Autodesk Inventor part; units mm, degrees
ref_plane "YZ Plane" through (0, 0, 0) normal (1, 0, 0) x (0, 1, 0)
ref_plane "XZ Plane" through (0, 0, 0) normal (0, 1, 0) x (-1, 0, 0)
ref_plane "XY Plane" through (0, 0, 0) normal (0, 0, 1) x (1, 0, 0)
sketch "Sketch1" plane through (0, 0, 0) normal (0, 0, 1) x (1, 0, 0)
  line L0 (-10, 4.2062) -> (5, 4.2062) construction
  line L1 (-10, -0.7938) -> (5, -0.7938)
  line L2 (5, 9.2062) -> (-10, 9.2062)
  arc A0 (-10, 9.2062) -> (-10, -0.7938) centre (-10, 4.2062) ccw
  arc A1 (5, -0.7938) -> (5, 9.2062) centre (5, 4.2062) ccw
  circle A2 centre (-2.5, 4.2062) radius 2.5
  point P0 (0, 0)
  dimension "d0" = 10
  dimension "d1" = 5
  dimension "d11" = 15
extrude "Extrusion3" add sketch "Sketch1" along normal blind 5 contours A0 L2 A1 L1 | A2
extrude "Extrusion4" add sketch "Sketch1" against normal blind 5 contours A2
properties material "Copper, Alloy"
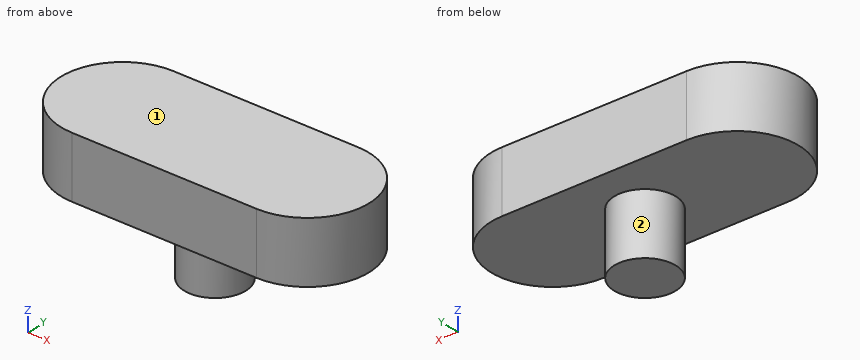
Source: CAD feature listing. Evaluate the final solid. Frame: model axes, mm. Face numbers are marked on the shaded views. A direction names the side the tool comes from. Give positions to 0.01 mm unless a question says otherwise; leave off trailing zeros. Loops run counter-clockwise (first coordinate to the right, second up) from the corner with the lowest first, then second, coordinate; pieces in that order, holes last. Notation, with made-up numbers: (36, 79) -> (40, 79) arc R17 cw to (40, 100) -> close; hole circle Ø11 at (5, 87). An arc over 180 degrees is marked (long way). Put each result on its own line as item: value. Start each with the question number.
1) Cut plane A-A (x = -2.5). Return loops of the section in (y, z), then the cut area to 3 significant figures.
2) Cut plane B-B (y = 5.5). Return loops of the section in (x, z).
3) Cut plane C-C (z = 1.75). Return loops of the section in (x, y), then the cut area to 3 significant figures.
4) Contact query for flat-ended pins moving along their axis: P1, Ø6, axis at x = -1, y = 7, coming from the -Z side; P2, Ø3, axis at y = 8, z = 3.5, coming from the -X side; P3, Ø5, axis at x = -8.5, y = 5.5, coming from the -Z side; P4, Ø1, axis at x = 6, z = 3.5, coming from the -Y side. Output: stop coordinate, or through.
5) Cut plane D-D (x = 2.5). Return loops of the section in (y, z), then the cut area to 3 significant figures.
6) Material intervals for probe 1 along Z at (x, y) = (-6.25, 7); probe 2 along Y at (x, z) = (-2.5, -3); probe 3 along X at (y, z) = (2.5, -3), sorted ascending.
7) Reachability of the marked faces 1 and 2 from +Z, -Z, +X, -X, +Y, -Y: full face, straight path, thin tool, end or side. Return the list, or none.
Results are:
1. outline: (-0.79, 0) -> (1.71, 0) -> (1.71, -5) -> (6.71, -5) -> (6.71, 0) -> (9.21, 0) -> (9.21, 5) -> (-0.79, 5) -> close
1. area: 75.0 mm2
2. outline: (-14.83, 0) -> (-4.64, 0) -> (-4.64, -5) -> (-0.36, -5) -> (-0.36, 0) -> (9.83, 0) -> (9.83, 5) -> (-14.83, 5) -> close
3. outline: (-10, -0.79) -> (5, -0.79) arc R5 ccw to (5, 9.21) -> (-10, 9.21) arc R5 ccw to start
3. area: 229 mm2
4. P1: stops at z = -5
4. P2: stops at x = -14.44
4. P3: stops at z = 0
4. P4: stops at y = -0.77
5. outline: (-0.79, 0) -> (9.21, 0) -> (9.21, 5) -> (-0.79, 5) -> close
5. area: 50.0 mm2
6. probe 1: z = 0 to 5
6. probe 2: y = 1.71 to 6.71
6. probe 3: x = -4.33 to -0.67
7. face 1: +Z, +X, -X, +Y, -Y
7. face 2: -Z
